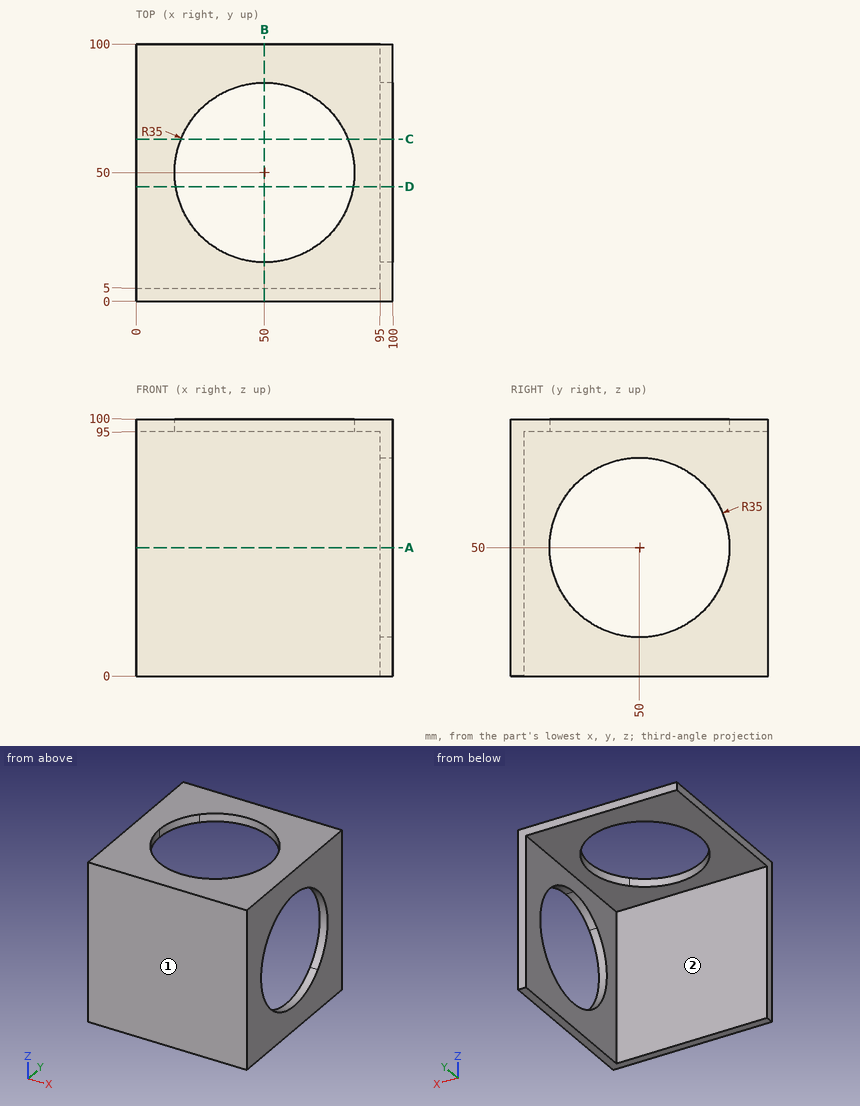
Here's the drawing with two shaded views (mm, measured from the low corner). I have some questions. A direction names the side the tool comes from. Coordinates: 2 decimals unless noted, no trailing zeros. Write each loop counter-clockwise with the first axis right and the second up, starting at its lowest first coordinate (ties: lowest second). Pieces come first, ordered by that corner, then holes. Notation, with made-up numbers: (45.25, -40) -> (91.25, -40) arc R9 cw to (91.25, -24) -> close; hole circle Ø9 at (36.5, 13). An arc over 180 degrees is marked (long way). Use a Markdown table: item, result. Add a question column.
(1) If we section it at D-D, the plane y = 44.5: Write out the boundary of the cut face in (x, z) (1 decimal), and give its area (3 significant figures).
(2) If we section it at B-B, the plane x = 50: Write out the boundary of the cut face in (y, z).
(3) If we section it at A-A, the plane z = 50: Write out the boundary of the cut face in (x, y).
(4) I'm going to push flat-ended pins straight in: P1, Ø3, axis at x = 64.5, y = 12, coming from the -Z side; P2, Ø3, axis at y = 67.5, z = 16.5, coming from the -X side; P3, Ø3, axis at x = 51.5, z = 79.5, coming from the +Y side. Where does each tip first touch, or does it pass through?
(5) Please list where these lines run through material, in increasing order: line 1 (Y direction, x = 55, z = 32.5); line 2 (Z direction, x = 11.5, y = 77).
(6) If we section it at C-C, the plane y = 63: Write out the boundary of the cut face in (x, z).
(7) For the marked faces 1 and 2, which set-ups out of +Z, -Z, +X, -X, +Y, -Y let a thin tool reach every point of the face, with its end or its side?
Outcome:
| question | item | result |
|---|---|---|
| 1 | outline | (0, 95) -> (15.4, 95) -> (15.4, 100) -> (0, 100) -> close; (84.6, 95) -> (95, 95) -> (95, 84.6) -> (100, 84.6) -> (100, 100) -> (84.6, 100) -> close; (95, 0) -> (100, 0) -> (100, 15.4) -> (95, 15.4) -> close |
| 1 | area | 284 mm^2 |
| 2 | outline | (0, 0) -> (5, 0) -> (5, 95) -> (15, 95) -> (15, 100) -> (0, 100) -> close; (85, 95) -> (100, 95) -> (100, 100) -> (85, 100) -> close |
| 3 | outline | (0, 0) -> (100, 0) -> (100, 15) -> (95, 15) -> (95, 5) -> (0, 5) -> close; (95, 85) -> (100, 85) -> (100, 100) -> (95, 100) -> close |
| 4 | P1 | stops at z = 95 |
| 4 | P2 | stops at x = 95 |
| 4 | P3 | stops at y = 5 |
| 5 | line 1 | y = 0 to 5 |
| 5 | line 2 | z = 95 to 100 |
| 6 | outline | (0, 95) -> (17.5, 95) -> (17.5, 100) -> (0, 100) -> close; (82.5, 95) -> (95, 95) -> (95, 82.5) -> (100, 82.5) -> (100, 100) -> (82.5, 100) -> close; (95, 0) -> (100, 0) -> (100, 17.5) -> (95, 17.5) -> close |
| 7 | face 1 | +Z, -Z, +X, -X, -Y |
| 7 | face 2 | -Z, -X, +Y |
